```python
from build123d import *

# Parameters (mm, degrees)
SKETCH1_W           = 50.8
SKETCH1_H           = 6.35
BOSS_EXTRUDE1_DEPTH = 137.16
SKETCH2_R           = 1.1303
CUT_EXTRUDE1_DEPTH  = 140.636485562


with BuildPart() as part:
    # Sketch1 → Boss-Extrude1 (new body)
    with BuildSketch(Plane(origin=(0, 0, 0), x_dir=(1, 0, 0), z_dir=(0, 1, 0))):
        Rectangle(SKETCH1_W, SKETCH1_H)
    extrude(amount=BOSS_EXTRUDE1_DEPTH)

    # Sketch2 → Cut-Extrude1 (cut, through all)
    with BuildSketch(Plane(origin=(0, 0, -3.175), x_dir=(-1, 0, 0), z_dir=(0, 0, -1))):
        with Locations((0, 128.27)):
            Circle(SKETCH2_R)
        with Locations(Location((0, 8.89, 0), (0, 0, 180))):
            Circle(SKETCH2_R)
    extrude(amount=-CUT_EXTRUDE1_DEPTH, mode=Mode.SUBTRACT)


solid = part.part
```
Verification items for the finished model (mm, model axes). Round coordinates to 2 decimals unless told otherwise and drop trailing zeros. Answer as a JSON object with one key per item and string values. Group by question number.
Q1. Thickness scan on line 1 (Y direction, x = 0, z = -0.5); line 2 (X direction, y = 8.89, z = -0.5); line 3 (Y direction, x = -1, z = -1.5). Record the ranges inside material, lowest first.
Q2. Mould release check, pull along Y, two halves, no side actions. Record for faces 1 (the flat face through (25.4, 68, 0)), 2 (the flat face through (0, 0, 0)), 3 (the cylindrical face through (0.245, 127.167, -0.044)): released by +Y, released by -Y, zero draft, split by the parting line, or undercut.
Q3. Go/stop test with a flat-tipped pin: pin 1 Ø2.5 at (x, y) = (0, 8.89) entering from -Z (3 decimals). Record where the tip stops, or that it passes through.
Found:
{
 "1": {"line 1": "y = 0 to 7.76, 10.02 to 127.14, 129.4 to 137.16", "line 2": "x = -25.4 to -1.13, 1.13 to 25.4", "line 3": "y = 0 to 8.36, 9.42 to 127.74, 128.8 to 137.16"},
 "2": {"face 1": "zero draft", "face 2": "released by -Y", "face 3": "undercut"},
 "3": {"pin 1": "stops at z = -3.175"}
}
